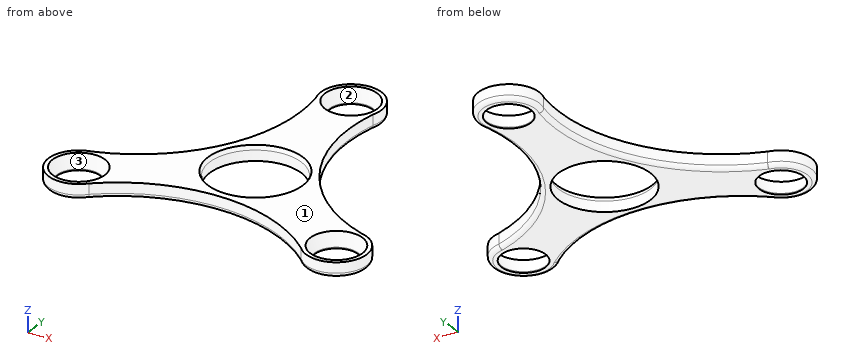
```python
from build123d import *

# Parameters (mm, degrees)
F0_R       = 5.25
F0_R_2     = 10.95
F1_DEPTH   = 3.5
F2_SIZE2   = 0.4
F2_SIZE    = 1
F3_SIZE2   = 1
F3_SIZE    = 3.2
F3_2_SIZE2 = 1
F3_2_SIZE  = 3.2
F3_3_SIZE2 = 1
F3_3_SIZE  = 3.2
F4_R       = 1


with BuildPart() as f1:
    # F0 (on Top) → F1 (new body)
    with BuildSketch(Plane.XY):
        with BuildLine():
            ThreePointArc((32.3008352617, -10.7570571715), (11.2405764073, 6.4897498146), (6.8345328504, 33.3518724858))
            ThreePointArc((6.8345328504, 33.3518724858), (0, 43.0208930969), (-6.8345328504, 33.3518724858))
            ThreePointArc((-6.8345328504, 33.3518724858), (-11.2405764073, 6.4897498146), (-32.3008352617, -10.7570571715))
            ThreePointArc((-32.3008352617, -10.7570571715), (-37.2571863154, -21.5104465485), (-25.4663024113, -22.5948153143))
            ThreePointArc((-25.4663024113, -22.5948153143), (0, -12.9794996293), (25.4663024113, -22.5948153143))
            ThreePointArc((25.4663024113, -22.5948153143), (37.2571863154, -21.5104465485), (32.3008352617, -10.7570571715))
        make_face()
        with Locations((-30.978502138, -17.8854465485)):
            Circle(F0_R, mode=Mode.SUBTRACT)
        with Locations((30.978502138, -17.8854465485)):
            Circle(F0_R, mode=Mode.SUBTRACT)
        Circle(F0_R_2, mode=Mode.SUBTRACT)
        with Locations((0, 35.7708930969)):
            Circle(F0_R, mode=Mode.SUBTRACT)
    extrude(amount=F1_DEPTH)

    # F2
    f2_edges = [f1.edges().sort_by_distance(p)[0] for p in [
        (-10.95, 0, 3.5),
    ]]
    f2_side = f1.faces().sort_by_distance((-10.95, 0, 1.75))[0]
    chamfer(f2_edges, length=F2_SIZE, length2=F2_SIZE2, reference=f2_side)

    # F3
    f3_edges = [f1.edges().sort_by_distance(p)[0] for p in [
        (-5.25, 35.770893, 3.5),
    ]]
    f3_side = f1.faces().sort_by_distance((-5.25, 35.770893, 1.75))[0]
    chamfer(f3_edges, length=F3_SIZE, length2=F3_SIZE2, reference=f3_side)

    # F3#2
    f3_2_edges = [f1.edges().sort_by_distance(p)[0] for p in [
        (-36.228502, -17.885447, 3.5),
    ]]
    f3_2_side = f1.faces().sort_by_distance((-36.228502, -17.885447, 1.75))[0]
    chamfer(f3_2_edges, length=F3_2_SIZE, length2=F3_2_SIZE2, reference=f3_2_side)

    # F3#3
    f3_3_edges = [f1.edges().sort_by_distance(p)[0] for p in [
        (25.728502, -17.885447, 3.5),
    ]]
    f3_3_side = f1.faces().sort_by_distance((25.728502, -17.885447, 1.75))[0]
    chamfer(f3_3_edges, length=F3_3_SIZE, length2=F3_3_SIZE2, reference=f3_3_side)

    # F4
    f4_edges = [f1.edges().sort_by_distance(p)[0] for p in [
        (0, -12.9795, 0),
        (11.240576, 6.48975, 0),
        (37.257186, -21.510447, 0),
        (0, 43.020893, 0),
        (-37.257186, -21.510447, 0),
        (-11.240576, 6.48975, 0),
    ]]
    fillet(f4_edges, radius=F4_R)


solid = f1.part
```
Read the model definition and answer for the solid it produces. Units are mm, in the model's axes. Face numbers are marked on the shaded views. Coordinates: 2 decimals unless noted, no trailing zeros. Order: outer loops, then holes, each group sorted by start corner. A loop starts at its lowest first (then second) coordinate and runs counter-clockwise, first axis right, second up. Notation, with made-up numbers: (34, 44.25) - (66, 44.25) arc R18 ccw to (66, 65.25) - close; hole circle Ø3 at (38, -13). An arc over 180 degrees is marked (long way). Answer as a JSON object with one key per item and string values. Group by question number.
Item 1: The mould has two halves that part along Y. Classify the marked faces 1, 2 and 3: +Y half, -Y half, draft (parallel to the pull), parting line (faces both ways), or undercut.
Item 2: Consider probe 1 along X at (y, z) = (-17, 2.6); probe 2 along X at (y, z) = (4.5, 1.85); probe 3 along Y at (x, z) = (-0.5, 3.05). Determine where each line is inside the solid, lowest interval first. Write a range as from..to.
Item 3: Flat-ended cylindrical pins translate along their axes: P1, Ø1.5, axis at y = -16.5, z = 0.5, coming from the +X side; P2, Ø6, axis at x = 6.5, y = -2, coming from the -Z side. Find the tip coordinate at first contact, or state that the pin passes through.
Item 4: Section A-A (x = 0) is taken. Give the vertices of the cut face in (y, z).
Results are:
{
 "1": {"face 1": "draft", "face 2": "undercut", "face 3": "undercut"},
 "2": {"probe 1": "x = -38.17..-36.88, -25.08..-17.14, 17.14..25.08, 36.88..38.17", "probe 2": "x = -12.47..-9.98, 9.98..12.47", "probe 3": "y = -12.98..-11.16, 11.16..29.68, 41.86..43"},
 "3": {"P1": "stops at x = 38.18", "P2": "passes through"},
 "4": {"outline": "(-12.98, 1) arc R1 ccw to (-11.98, 0) - (-10.95, 0) - (-10.95, 2.5) - (-11.35, 3.5) - (-12.98, 3.5) - close; (10.95, 0) - (30.52, 0) - (30.52, 0.3) - (29.52, 3.5) - (11.35, 3.5) - (10.95, 2.5) - close; (41.02, 0) - (42.02, 0) arc R1 ccw to (43.02, 1) - (43.02, 3.5) - (42.02, 3.5) - (41.02, 0.3) - close"}
}
